Geometry check sheet. Reference: the model listing, model coordinates, mm. A direction names the side the tool comes from. Coordinates: 2 decimals unless noted, no trailing zeros. Write each loop counter-clockwise with the first axis right and the second up, starting at its lowest first coordinate (ties: lowest second). Pieces come first, ordered by that corner, then holes. Notation, with made-up numbers: (4.5, -36.5) -> (49.5, -36.5) arc R31 cw to (49.5, 2.5) -> close; hole circle Ø3 at (49.25, 29.25). An arc over 180 degrees is marked (long way). Answer as CSV lines item,"result".
```python
from build123d import *

# Parameters (mm, degrees)
BOSS_EXTRU_1_DEPTH = 5


with BuildPart() as part:
    # Esquisse1 → Boss.-Extru.1 (new body)
    with BuildSketch(Plane(origin=(0, 0, 0), x_dir=(0, 0, -1), z_dir=(1, 0, 0))):
        Polygon((20.428249593, -55.741422484), (-13.843425106, -75.528183097), (-58.387612711, 1.624613017), (-58.387612711, 11.624613017), (-63.387612711, 11.624613017), (-63.387612711, 21.624613017), (-58.387612711, 21.624613017), (-58.387612711, 31.624613017), (7.224475537, 38.834467888), (8.438400995, 33.984067391), (30.488285558, 39.502563492), (29.2743601, 44.352963989), (38.975161094, 46.780814906), (40.189086552, 41.930414409), (49.889887546, 44.358265326), (68.059646801, -28.241422484), (29.08850363, -50.741422484), (31.58850363, -55.071549503), (22.928249593, -60.071549503), align=None)
        with BuildLine():
            Line((-11.75, 23), (11.75, 23))
            ThreePointArc((11.75, 23), (20.058504679, 19.558504679), (23.5, 11.25))
            Line((23.5, 11.25), (23.5, -11.25))
            ThreePointArc((23.5, -11.25), (20.058504679, -19.558504679), (11.75, -23))
            Line((11.75, -23), (-11.75, -23))
            ThreePointArc((-11.75, -23), (-20.058504679, -19.558504679), (-23.5, -11.25))
            Line((-23.5, -11.25), (-23.5, 11.25))
            ThreePointArc((-23.5, 11.25), (-20.058504679, 19.558504679), (-11.75, 23))
        make_face(mode=Mode.SUBTRACT)
    extrude(amount=BOSS_EXTRU_1_DEPTH)


solid = part.part
```
Item 1: Cross-section at C-C, the plane z = 20. Record the cut outline in (x, y).
Responses:
outline,"(0, -64.86) -> (5, -64.86) -> (5, -19.62) -> (0, -19.62) -> close; (0, 19.62) -> (5, 19.62) -> (5, 35.84) -> (0, 35.84) -> close"
Item 2: Cross-section at D-D, the plane z = 44. Record the cut outline in (x, y), plus the area to 3 significant figures.
Responses:
outline,"(0, -23.3) -> (5, -23.3) -> (5, 33.21) -> (0, 33.21) -> close"
area,"283 mm2"
Item 3: Cross-section at B-B, the plane y = -0.5. Record the cut outline in (x, z), plus the area to 3 significant figures.
Responses:
outline,"(0, -61.12) -> (5, -61.12) -> (5, -23.5) -> (0, -23.5) -> close; (0, 23.5) -> (5, 23.5) -> (5, 57.16) -> (0, 57.16) -> close"
area,"356 mm2"
Item 4: Set-up check for faces 1 (the flat face through (2.465, -57.937, -21.696)), 2 (the cylindrical face through (2.465, -19.467, -20.149)), 3 (the flat face through (2, 21.625, 61)): record each of +Z, -Z, +X, -X, +Y, -Y from which the full face is reachable in a straight line by a thin tool's end or side.
Responses:
face 1,"+X, -X, -Y"
face 2,"+X, -X"
face 3,"+Z, +X, -X, +Y"
Item 5: Thickness scan on probe 1 along Z at (x, y) = (4.8, 14); probe 2 along Y at (x, z) = (1, 14.5); probe 3 along Y at (x, z) = (2.25, 17.5). Record the ranges inside material, lowest first.
Responses:
probe 1,"z = -57.49 to -23.17, 23.17 to 63.39"
probe 2,"y = -74.39 to -22.67, 22.67 to 36.45"
probe 3,"y = -69.19 to -21.5, 21.5 to 36.12"
Item 6: Release check for a two-part mould opening along Z. For faces 4 (the flat face through (2, 7, 58.388)), 5 (the flat face through (0, -27, -3)), 6 (the flat face through (2, -23, 0)) record: +Z half, -Z half, draft (parallel to the pull), parting line (faces both ways), or undercut.
Responses:
face 4,"+Z half"
face 5,"draft"
face 6,"undercut"
Item 7: Cross-section at A-A, the plane x = 3.25. Record the cut outline in (y, z).
Responses:
outline,"(-75.53, 13.84) -> (-55.74, -20.43) -> (-60.07, -22.93) -> (-55.07, -31.59) -> (-50.74, -29.09) -> (-28.24, -68.06) -> (44.36, -49.89) -> (41.93, -40.19) -> (46.78, -38.98) -> (44.35, -29.27) -> (39.5, -30.49) -> (33.98, -8.44) -> (38.83, -7.22) -> (31.62, 58.39) -> (21.62, 58.39) -> (21.62, 63.39) -> (11.62, 63.39) -> (11.62, 58.39) -> (1.62, 58.39) -> close; hole (-23, -11.75) arc R11.75 ccw to (-11.25, -23.5) -> (11.25, -23.5) arc R11.75 ccw to (23, -11.75) -> (23, 11.75) arc R11.75 ccw to (11.25, 23.5) -> (-11.25, 23.5) arc R11.75 ccw to (-23, 11.75) -> close"
Item 8: Depth check by flat-ended pin: pin 1 Ø2 at (x, y) = (1.5, -15) entering from +Z; pin 2 Ø2.5 at (x, z) = (1.5, 61.5) entering from -Y; pin 3 Ø2.5 at (x, z) = (3.5, 2) entering from +Y; pin 4 Ø2 at (y, z) = (-47, 18.5) entering from -X. Enter the tip coordinate at first touch or a pass-through.
Responses:
pin 1,"stops at z = 49.37"
pin 2,"stops at y = 11.62"
pin 3,"stops at y = 37.96"
pin 4,"stops at x = 0"
